Build history of the part. All positions in model axes, mm. A direction names the side the tool comes from. Round coordinates to 2 decimals unless told otherwise and drop trailing zeros. Write each loop counter-clockwise with the first axis right and the second up, starting at its lowest first coordinate (ties: lowest second). Pieces come first, ordered by that corner, then holes.
Item 1: Wall check: probe 1 along Z at (x, y) = (3, -7); probe 2 along X at (y, z) = (-6.75, 16). Give the ranges that are in metal, low to high.
Item 2: Drop a flat-ended pin along its axis: pin 1 Ø4 at (y, z) = (-6, 21) entering from -X. Give the stop position or say it passes through.
Item 3: Band-saw the part on B-B, the plane y = -3.75. Write the cut outline in (x, z), then the cut area to 3 significant figures.
Item 4: Band-saw the part on A-A, the plane x = 35. Write the cut outline in (y, z), then the cut area to 3 significant figures.
Item 5: Band-saw the part on C-C, the plane z = 19. Write the cut outline in (x, y).
Item 6: 3-axis set-ups, long thin cutter, end or side, ignore diameter. For faces 1 (the flat face through (31.75, -6, 19)), 2 (the flat face through (6, -6, 25.4)), 3 (the flat face through (44.45, -6, 6)): which of +Z, -Z, +X, -X, +Y, -Y reach the whole face in a straight line?
```python
from build123d import *

# Parameters (mm, degrees)
F1_DEPTH = 12.7


with BuildPart() as f1:
    # F0 (on Front) → F1 (new body)
    with BuildSketch(Plane.XZ):
        Polygon((0, 12.7), (0, 0), (44.45, 0), (44.45, 12.7), (31.75, 12.7), (31.75, 25.4), (44.45, 25.4), (44.45, 38.1), (0, 38.1), (0, 25.4), (12.7, 25.4), (12.7, 12.7), align=None)
    extrude(amount=F1_DEPTH)


solid = f1.part
```
Results:
1. probe 1: z = 0 to 12.7, 25.4 to 38.1
1. probe 2: x = 12.7 to 31.75
2. pin 1: stops at x = 12.7
3. outline: (0, 0) - (44.45, 0) - (44.45, 12.7) - (31.75, 12.7) - (31.75, 25.4) - (44.45, 25.4) - (44.45, 38.1) - (0, 38.1) - (0, 25.4) - (12.7, 25.4) - (12.7, 12.7) - (0, 12.7) - close
3. area: 1,370 mm2
4. outline: (-12.7, 0) - (0, 0) - (0, 12.7) - (-12.7, 12.7) - close; (-12.7, 25.4) - (0, 25.4) - (0, 38.1) - (-12.7, 38.1) - close
4. area: 323 mm2
5. outline: (12.7, -12.7) - (31.75, -12.7) - (31.75, 0) - (12.7, 0) - close
6. face 1: +X, +Y, -Y
6. face 2: -X, +Y, -Y
6. face 3: +Z, -Z, +X, +Y, -Y
